```python
from build123d import *

# Parameters (mm, degrees)
F0_W      = 38.1
F0_H      = 38.1
F1_DEPTH  = 38.1
F6_DEPTH  = 38.1
F8_DEPTH  = 38.1
F9_W      = 25.4
F9_H      = 7.62
F10_DEPTH = 38.1


with BuildPart() as f1:
    # F0 (on Front) → F1 (new body)
    with BuildSketch(Plane.XZ):
        with Locations((19.05, 19.05)):
            Rectangle(F0_W, F0_H)
    extrude(amount=F1_DEPTH)

    # F5 (on offset) → F6 (cut)
    with BuildSketch(Plane.YZ.offset(38.1)):
        Polygon((-11.43, 15.875), (-6.35, 38.1), (-31.75, 38.1), (-26.67, 15.875), (-21.59, 28.575), (-16.51, 28.575), align=None)
        Polygon((-38.1, 0), (-31.75, 0), (-38.1, 38.1), align=None)
        Polygon((-25.4, 0), (-12.7, 0), (-19.05, 15.875), align=None)
        Polygon((-6.35, 0), (0, 0), (0, 38.1), align=None)
    extrude(amount=-F6_DEPTH, mode=Mode.SUBTRACT)

    # F7 (on offset) → F8 (cut)
    with BuildSketch(Plane.XZ.offset(38.1)):
        Polygon((0, 38.1), (0, 0), (6.35, 38.1), align=None)
        Polygon((25.4, 38.1), (12.7, 38.1), (19.05, 22.225), align=None)
        Polygon((31.75, 38.1), (38.1, 0), (38.1, 38.1), align=None)
        Polygon((11.43, 22.025449), (6.35, 0), (31.75, 0), (26.67, 21.632593), (21.59, 9.525), (16.51, 9.525), align=None)
    extrude(amount=-F8_DEPTH, mode=Mode.SUBTRACT)

    # F9 (on offset) → F10 (cut)
    with BuildSketch(Plane.XY.offset(38.1)):
        with Locations((25.4, -11.43)):
            Rectangle(F9_W, F9_H)
        with Locations((12.7, -26.67)):
            Rectangle(F9_W, F9_H)
    extrude(amount=-F10_DEPTH, mode=Mode.SUBTRACT)


solid = f1.part
```
The listing builds one solid part. Answer for the finished solid, in the listing's coordinates (mm). A direction names the side the tool comes from. Coordinates: 2 decimals unless noted, no trailing zeros. Loops run counter-clockwise (first coordinate to the right, second up) from the corner with the lowest first, then second, coordinate; pieces in that order, holes last. Notation, with made-up numbers: M 20,80.5 L 74,80.5 A15 cw 74,102.5 Z; hole C -36.75,51.5 d6. An arc over 180 degrees is marked long. Answer as a JSON object with one key per item and string values. Group by question number.
Item 1: Section B-B (x = 29.5) is taken. Write down the section's boundary in (y, z) (3 decimals).
Item 2: Section C-C (x = 18.5) is taken. Give the number of separate pieces and of enclosed holes in the cut face, and give its area (3 significant figures).
Item 3: Consider L1, parallel to Y at x = 19.5, z = 14; L2, parallel to X at y = -31.5, z = 12; L3, parallel to Y at x = 2.5, z = 7. Determine where each line is inside the solid, lowest interval first.
Item 4: Section A-A (z = 28) is taken. Write down the section's boundary in (x, y).
Item 5: Section D-D (y = -8.5) is taken. Write down the section's boundary in (x, z).
Item 6: Which of the six approach directions +Z, -Z, +X, -X, +Y, -Y give full straight-line access (tool end or side, diameter ignored) to faces 4 (the face through (22.2, -33.5, 30.1)), 5 (the face through (29.675, -24.166, 22.136)), 6 (the face through (5.08, -15.83, 7.83))?
Item 7: Each of these flat-tipped pins is pushed along its axis until it touches: P1, Ø5, axis at y = -22, z = 8, coming from the +X side; P2, Ø15, axis at x = 20, z = 15, coming from the +Y side; P3, Ø8, axis at x = 6, z = 31, coming from the +Y side; P4, Ø3, axis at x = 8, y = -27.5, coming from the +Z side. Where does it stop, or does it pass through?
Item 8: Determine the mould class of faces 1 (the face through (9.49, -32.44, 13.61)), 2 (the face through (6, -21, 11)), 3 (the face through (3.13, -9.05, 18.78)) for opening direction X: +X half, -X half, draft (parallel to the pull), parting line (faces both ways), or undercut.
Solved:
{
 "1": {"outline": "M -38.1,38.1 L -33.347,9.581 L -21.567,9.581 L -19.05,15.875 L -16.533,9.581 L -15.24,9.581 L -15.24,25.4 L -16.51,28.575 L -21.59,28.575 L -26.67,15.875 L -31.75,38.1 Z; M -7.62,9.581 L -4.753,9.581 L 0,38.1 L -6.35,38.1 L -7.62,32.544 Z"},
 "2": {"separate pieces": "3", "enclosed holes": "0", "area": "205 mm2"},
 "3": {"L1": "y = -34.08 to -30.48, -22.86 to -19.8, -18.3 to -15.24, -7.62 to -4.02", "L2": "x = 2 to 9.12, 15.5 to 22.63, 28.93 to 36.1", "L3": "y = -32.92 to -30.48, -22.86 to -22.6, -15.5 to -5.18"},
 "4": {"outline": "M 4.67,-36.42 L 16.74,-36.42 L 16.74,-30.48 L 4.67,-30.48 Z; M 4.67,-21.82 L 16.74,-21.82 L 16.74,-16.28 L 4.67,-16.28 Z; M 4.67,-8.66 L 12.7,-8.66 L 12.7,-7.62 L 16.74,-7.62 L 16.74,-1.68 L 4.67,-1.68 Z; M 21.36,-36.42 L 33.43,-36.42 L 33.43,-29.44 L 25.4,-29.44 L 25.4,-30.48 L 21.36,-30.48 Z; M 21.36,-21.82 L 33.43,-21.82 L 33.43,-16.28 L 21.36,-16.28 Z; M 21.36,-7.62 L 33.43,-7.62 L 33.43,-1.68 L 21.36,-1.68 Z"},
 "5": {"outline": "M 0,0 L 6.35,0 L 11.43,22.03 L 12.7,18.9 L 12.7,28.69 L 4.78,28.69 Z"},
 "6": {"face 4": "+Z, +Y, -Y", "face 5": "+Z, +X, -X", "face 6": "-Z, +X, -X"},
 "7": {"P1": "stops at x = 37.14", "P2": "stops at y = -2.6", "P3": "stops at y = -0.52", "P4": "passes through"},
 "8": {"face 1": "undercut", "face 2": "draft", "face 3": "-X half"}
}
